Here's how the part is built. I have some questions about the finished solid (model axes, mm). A direction names the side the tool comes from. Round coordinates to 2 decimals unless told otherwise and drop trailing zeros. Loops run counter-clockwise (first coordinate to the right, second up) from the corner with the lowest first, then second, coordinate; pieces in that order, holes last. Notation, with made-up numbers: M 27,68.25 L 82,68.25 A31 ccw 82,105.25 Z; hole C 69,-21 d3. An arc over 180 degrees is marked long. Answer as CSV lines item,"result".
```python
from build123d import *

# Parameters (mm, degrees)
SKETCH_1_W          = 70
SKETCH_1_H          = 70
EXTRUDE_1_DEPTH     = 19
SKETCH_2_R          = 22.8
CUT_EXTRUDE_1_DEPTH = 8.8
SKETCH_3_R          = 1.5
CUT_EXTRUDE_2_DEPTH = 19
SKETCH_5_R          = 3.25
CUT_EXTRUDE_3_DEPTH = 2
SKETCH_6_R          = 3.1
CUT_EXTRUDE_4_DEPTH = 7.5
CHAMFER_2_SIZE      = 0.5
CUT_EXTRUDE_5_DEPTH = 3
FILLET_1_R          = 10


with BuildPart() as part:
    # Эскиз1 → Бобышка-Вытянуть1 (new body)
    with BuildSketch(Plane.XY):
        Rectangle(SKETCH_1_W, SKETCH_1_H)
    extrude(amount=EXTRUDE_1_DEPTH)

    # Эскиз2 → Вырез-Вытянуть1 (cut)
    with BuildSketch(Plane.XY.offset(19)):
        Circle(SKETCH_2_R)
    extrude(amount=-CUT_EXTRUDE_1_DEPTH, mode=Mode.SUBTRACT)

    # Эскиз3 → Вырез-Вытянуть2 (cut)
    with BuildSketch(Plane.XY.offset(19)):
        with Locations((-8.343458848, 25.67852594)):
            Circle(SKETCH_3_R)
        with Locations((8.343458848, 25.67852594)):
            Circle(SKETCH_3_R)
        with Locations((15.870201812, 21.843458848)):
            Circle(SKETCH_3_R)
        with Locations((21.843458848, 15.870201812)):
            Circle(SKETCH_3_R)
        with Locations((25.67852594, 8.343458848)):
            Circle(SKETCH_3_R)
        with Locations((25.67852594, -8.343458848)):
            Circle(SKETCH_3_R)
        with Locations((21.843458848, -15.870201812)):
            Circle(SKETCH_3_R)
        with Locations((15.870201812, -21.843458848)):
            Circle(SKETCH_3_R)
        with Locations((8.343458848, -25.67852594)):
            Circle(SKETCH_3_R)
        with Locations((-8.343458848, -25.67852594)):
            Circle(SKETCH_3_R)
        with Locations((-15.870201812, -21.843458848)):
            Circle(SKETCH_3_R)
        with Locations((-21.843458848, -15.870201812)):
            Circle(SKETCH_3_R)
        with Locations((-25.67852594, -8.343458848)):
            Circle(SKETCH_3_R)
        with Locations((-25.67852594, 8.343458848)):
            Circle(SKETCH_3_R)
        with Locations((-21.843458848, 15.870201812)):
            Circle(SKETCH_3_R)
        with Locations((-15.870201812, 21.843458848)):
            Circle(SKETCH_3_R)
    extrude(amount=-CUT_EXTRUDE_2_DEPTH, mode=Mode.SUBTRACT)

    # Эскиз5 → Вырез-Вытянуть3 (cut)
    with BuildSketch(Plane(origin=(0, 0, 0), x_dir=(-1, 0, 0), z_dir=(0, 0, -1))):
        with Locations((-8.343458848, 25.67852594)):
            Circle(SKETCH_5_R)
        with Locations((8.343458848, 25.67852594)):
            Circle(SKETCH_5_R)
        with Locations((15.870201812, 21.843458848)):
            Circle(SKETCH_5_R)
        with Locations((21.843458848, 15.870201812)):
            Circle(SKETCH_5_R)
        with Locations((25.67852594, 8.343458848)):
            Circle(SKETCH_5_R)
        with Locations((25.67852594, -8.343458848)):
            Circle(SKETCH_5_R)
        with Locations((21.843458848, -15.870201812)):
            Circle(SKETCH_5_R)
        with Locations((15.870201812, -21.843458848)):
            Circle(SKETCH_5_R)
        with Locations((8.343458848, -25.67852594)):
            Circle(SKETCH_5_R)
        with Locations((-8.343458848, -25.67852594)):
            Circle(SKETCH_5_R)
        with Locations((-15.870201812, -21.843458848)):
            Circle(SKETCH_5_R)
        with Locations((-21.843458848, -15.870201812)):
            Circle(SKETCH_5_R)
        with Locations((-25.67852594, -8.343458848)):
            Circle(SKETCH_5_R)
        with Locations((-25.67852594, 8.343458848)):
            Circle(SKETCH_5_R)
        with Locations((-21.843458848, 15.870201812)):
            Circle(SKETCH_5_R)
        with Locations((-15.870201812, 21.843458848)):
            Circle(SKETCH_5_R)
    extrude(amount=-CUT_EXTRUDE_3_DEPTH, mode=Mode.SUBTRACT)

    # Эскиз6 → Вырез-Вытянуть4 (cut)
    with BuildSketch(Plane(origin=(0, 0, 0), x_dir=(-1, 0, 0), z_dir=(0, 0, -1))):
        with Locations((0, -19)):
            Circle(SKETCH_6_R)
        with Locations((0, 19)):
            Circle(SKETCH_6_R)
        with Locations((-19, 0)):
            Circle(SKETCH_6_R)
        with Locations((19, 0)):
            Circle(SKETCH_6_R)
        Circle(SKETCH_6_R)
    extrude(amount=-CUT_EXTRUDE_4_DEPTH, mode=Mode.SUBTRACT)

    # Фаска2
    chamfer_2_edges = [part.edges().sort_by_distance(p)[0] for p in [
        (-22.8, 0, 10.2),
    ]]
    chamfer(chamfer_2_edges, length=CHAMFER_2_SIZE)

    # Эскиз7 → Вырез-Вытянуть5 (cut)
    with BuildSketch(Plane.XY.offset(10.2)):
        Polygon((-2.973353886, 5.15), (-5.946707773, 0), (-2.973353886, -5.15), (2.973353886, -5.15), (5.946707773, 0), (2.973353886, 5.15), align=None)
    extrude(amount=-CUT_EXTRUDE_5_DEPTH, mode=Mode.SUBTRACT)

    # Скругление1
    fillet_1_edges = [part.edges().sort_by_distance(p)[0] for p in [
        (35, -35, 9.5),
        (-35, -35, 9.5),
        (-35, 35, 9.5),
        (35, 35, 9.5),
    ]]
    fillet(fillet_1_edges, radius=FILLET_1_R)


solid = part.part
```
1. If I drill on line 1 (Y direction, x = 24.5, z = 11); line 2 (Y direction, x = 0.5, z = 13); line 3 (Y direction, x = -7, z = 17.5), over which ranges is the centre line in solid material (lowest first)? Write a range as [from, to].
Evaluation:
line 1,"y = [-35, -9.27], [-7.42, 7.42], [9.27, 35]"
line 2,"y = [-35, -22.79], [22.79, 35]"
line 3,"y = [-35, -26.35], [-25.01, -21.7], [21.7, 25.01], [26.35, 35]"
2. I want a section at B-B, the plane z = 15. Count the separate pieces of the cut face and the enclosed holes in it, and give its area (3 significant figures).
Evaluation:
separate pieces,"1"
enclosed holes,"17"
area,"3,070 mm²"
3. We'd pull the mould along X, two halves only. Please class faces 1 (the flat face through (0, 35, 9)), 2 (the flat face through (-14, -23, 2)), 3 (the cylindrical face through (-32.15, -31.99, 9.63)): pulls with the +X half, pulls with the -X half, needs draft (parallel to the pull), parting line crosses it, or undercut.
Evaluation:
face 1,"needs draft"
face 2,"undercut"
face 3,"pulls with the -X half"
4. Which directions (+Z, -Z, +X, -X, +Y, -Y) give clear straight access to the entire face, cutting with the end or side of a thin tool? Please do faces 4 (the cylindrical face through (24.239, 18.067, 0.986)), 5 (the cylindrical face through (-6.958, -26.253, 10.619)), 6 (the flat face through (4.44, -2.61, 8.72)).
Evaluation:
face 4,"-Z"
face 5,"+Z, -Z"
face 6,"+Z"
5. I want a section at D-D, the plane y = 30. Please give me the cut outline in (x, z), and give its area (3 significant figures).
Evaluation:
outline,"M -33.66,0 L 33.66,0 L 33.66,19 L -33.66,19 Z"
area,"1,280 mm²"
6. For P1, Ø5, axis at x = 0, y = 19, coming from the -Z side; P2, Ø1.9, axis at x = 22, y = 17, coming from the -Z side; P3, Ø2.5, axis at x = 21.84, y = -15.87, coming from the +Z side; P4, Ø2, axis at y = 27.5, z = 14.5, coming from the -X side, each with a flat end and sliding along its axis, tell me the tip position at first contact or that it passes through.
Evaluation:
P1,"stops at z = 7.5"
P2,"stops at z = 2"
P3,"passes through"
P4,"stops at x = -34.89"
7. I want a section at A-A, the plane x = 0. Please give me the cut outline in (y, z).
Evaluation:
outline,"M -35,0 L -22.1,0 L -22.1,7.5 L -15.9,7.5 L -15.9,0 L -3.1,0 L -3.1,7.2 L -5.15,7.2 L -5.15,10.2 L -22.3,10.2 L -22.8,10.7 L -22.8,19 L -35,19 Z; M 3.1,0 L 15.9,0 L 15.9,7.5 L 22.1,7.5 L 22.1,0 L 35,0 L 35,19 L 22.8,19 L 22.8,10.7 L 22.3,10.2 L 5.15,10.2 L 5.15,7.2 L 3.1,7.2 Z"
